Geometry: final body of the model. Coordinates: model frame, mm. Round coordinates to 2 decimals unless told otherwise and drop trailing zeros. Loops run counter-clockwise (first coordinate to the right, second up) from the corner with the lowest first, then second, coordinate; pieces in that order, holes last. Notation, with made-up numbers: (8.5, 38.25) - (36.5, 38.25) arc R16 cw to (36.5, 52.25) - close; hole circle Ø6 at (78.25, 33). An arc over 180 degrees is marked (long way). Answer in a Markdown table with one row per item. Add a question column.
from build123d import *

# Parameters (mm, degrees)
ESQUISSE1_R             = 47.5
BOSS_EXTRU_1_DEPTH      = 10
ESQUISSE3_W             = 100
ESQUISSE3_H             = 10
ENL_V_MAT_EXTRU_1_DEPTH = 11
ESQUISSE4_R             = 2.5
ENL_V_MAT_EXTRU_2_DEPTH = 11
ESQUISSE6_W             = 150
ESQUISSE6_H             = 120
BOSS_EXTRU_2_DEPTH      = 10
ESQUISSE7_W             = 10
ESQUISSE7_H             = 50
ESQUISSE7_W_2           = 50
ESQUISSE7_H_2           = 9.570800355
ENL_V_MAT_EXTRU_3_DEPTH = 10


with BuildPart() as part:
    # Esquisse1 → Boss.-Extru.1 (new body)
    with BuildSketch(Plane.XY):
        Polygon((-310, -75.642859016), (0, 414.561180135), (310, -75.642859016), align=None)
        with Locations((-157.5, 0)):
            Circle(ESQUISSE1_R, mode=Mode.SUBTRACT)
        with Locations((-52.5, 0)):
            Circle(ESQUISSE1_R, mode=Mode.SUBTRACT)
        with Locations((52.5, 0)):
            Circle(ESQUISSE1_R, mode=Mode.SUBTRACT)
        with Locations((157.5, 0)):
            Circle(ESQUISSE1_R, mode=Mode.SUBTRACT)
        with Locations((-105, 90.932667397)):
            Circle(ESQUISSE1_R, mode=Mode.SUBTRACT)
        with Locations((0, 90.932667397)):
            Circle(ESQUISSE1_R, mode=Mode.SUBTRACT)
        with Locations((105, 90.932667397)):
            Circle(ESQUISSE1_R, mode=Mode.SUBTRACT)
        with Locations((-52.5, 181.865334795)):
            Circle(ESQUISSE1_R, mode=Mode.SUBTRACT)
        with Locations((52.5, 181.865334795)):
            Circle(ESQUISSE1_R, mode=Mode.SUBTRACT)
        with Locations((0, 272.798002192)):
            Circle(ESQUISSE1_R, mode=Mode.SUBTRACT)
    extrude(amount=BOSS_EXTRU_1_DEPTH)

    # Esquisse3 → Enlèv. mat.-Extru.1 (cut, through all)
    with BuildSketch(Plane.XY.offset(10)):
        Polygon((-269.913793103, -12.254405678), (-261.461999325, -17.599233264), (-208.013723463, 66.918704521), (-216.465517241, 72.263532107), align=None)
        Polygon((-181.724137931, 127.200191667), (-173.272344153, 121.855364081), (-119.82406829, 206.373301865), (-128.275862069, 211.718129452), align=None)
        Polygon((-93.534482759, 266.654789012), (-85.08268898, 261.309961425), (-31.634413118, 345.82789921), (-40.086206897, 351.172726796), align=None)
        Polygon((269.913793103, -12.254405678), (261.461999325, -17.599233264), (208.013723463, 66.918704521), (216.465517241, 72.263532107), align=None)
        Polygon((181.724137931, 127.200191667), (173.272344153, 121.855364081), (119.82406829, 206.373301865), (128.275862069, 211.718129452), align=None)
        Polygon((93.534482759, 266.654789012), (85.08268898, 261.309961425), (31.634413118, 345.82789921), (40.086206897, 351.172726796), align=None)
        with Locations((-160, -70.642859016)):
            Rectangle(ESQUISSE3_W, ESQUISSE3_H)
        with Locations((160, -70.642859016)):
            Rectangle(ESQUISSE3_W, ESQUISSE3_H)
    extrude(amount=-ENL_V_MAT_EXTRU_1_DEPTH, mode=Mode.SUBTRACT)

    # Esquisse4 → Enlèv. mat.-Extru.2 (cut, through all)
    with BuildSketch(Plane.XY.offset(10)):
        with Locations((-157.5, -55.642859016)):
            Circle(ESQUISSE4_R)
        with Locations((-52.5, -55.642859016)):
            Circle(ESQUISSE4_R)
        with Locations((52.5, -55.642859016)):
            Circle(ESQUISSE4_R)
        with Locations((157.5, -55.642859016)):
            Circle(ESQUISSE4_R)
        with Locations((-105, 29.047375097)):
            Circle(ESQUISSE4_R)
        with Locations((0, 29.047375097)):
            Circle(ESQUISSE4_R)
        with Locations((105, 29.047375097)):
            Circle(ESQUISSE4_R)
        with Locations((-52.5, 119.980042494)):
            Circle(ESQUISSE4_R)
        with Locations((52.5, 119.980042494)):
            Circle(ESQUISSE4_R)
        with Locations((0, 210.912709891)):
            Circle(ESQUISSE4_R)
    extrude(amount=-ENL_V_MAT_EXTRU_2_DEPTH, mode=Mode.SUBTRACT)

    # Esquisse6 → Boss.-Extru.2 (add)
    with BuildSketch(Plane.XY.offset(10)):
        with Locations((0, -135.642859016)):
            Rectangle(ESQUISSE6_W, ESQUISSE6_H)
    extrude(amount=-BOSS_EXTRU_2_DEPTH)

    # Esquisse7 → Enlèv. mat.-Extru.3 (cut)
    with BuildSketch(Plane.XY.offset(10)):
        with Locations((-70, -135.642859016)):
            Rectangle(ESQUISSE7_W, ESQUISSE7_H)
        with Locations((0, -190.857458839)):
            Rectangle(ESQUISSE7_W_2, ESQUISSE7_H_2)
        with Locations((70, -135.642859016)):
            Rectangle(ESQUISSE7_W, ESQUISSE7_H)
    extrude(amount=-ENL_V_MAT_EXTRU_3_DEPTH, mode=Mode.SUBTRACT)


solid = part.part
1) Section D-D, the plane y = 373.5. Return the cut outline in (x, z).
2) Section A-A, the plane y = 0. Return the cut outline in (x, z).
3) Pull-direction query (Y, two-part tool) for faces 1 (the flat face through (1, 20, 10)), 2 (the flat face through (198.85, 100.12, 4.93)), 3 (the cylindrical face through (147.2, -46.37, 4.93)), 4 (the cylindrical face through (-10.297, 44.562, 4.93)); classes: pulls with the +Y half, pulls with the -Y half, needs draft (parallel to the pull), parting line crosses it, or undercut.
4) Contact query for flat-ended pins moving along their axis: pin 1 Ø5 at (x, z) = (235.5, 5.5) entering from -Y; pin 2 Ø5 at (x, z) = (-123.5, 4.5) entering from -Y; pin 3 Ø3 at (y, z) = (-72.5, 6.5) entering from -X. Output: stop coordinate, or through.
5) Material intervals for line 1 along X through (y, z) = (-74, 7); line 2 along Y through (x, z) = (-122, 6.25); line 3 along Y through (x, z) = (-52.5, 3), sorted ascending. Write a range as from..to.
6) Section B-B, the plane y = 194.5. Return the cut outline in (x, z).
7) Section C-C, the plane y = -91. Return the cut outline in (x, z), and give its area (3 significant figures).
Evaluation:
| question | item | result |
|---|---|---|
| 1 | outline | (-25.97, 0) - (25.97, 0) - (25.97, 10) - (-25.97, 10) - close |
| 2 | outline | (-250.33, 0) - (-205, 0) - (-205, 10) - (-250.33, 10) - close; (-110, 0) - (-100, 0) - (-100, 10) - (-110, 10) - close; (-5, 0) - (5, 0) - (5, 10) - (-5, 10) - close; (100, 0) - (110, 0) - (110, 10) - (100, 10) - close; (205, 0) - (250.33, 0) - (250.33, 10) - (205, 10) - close |
| 3 | face 1 | needs draft |
| 3 | face 2 | pulls with the +Y half |
| 3 | face 3 | undercut |
| 3 | face 4 | undercut |
| 4 | pin 1 | stops at y = -75.64 |
| 4 | pin 2 | stops at y = -65.64 |
| 4 | pin 3 | stops at x = -308.96 |
| 5 | line 1 | x = -308.96..-210, -110..110, 210..308.96 |
| 5 | line 2 | y = -65.64..-31.56, 31.56..46.58, 135.29..202.93, 207.75..221.64 |
| 5 | line 3 | y = -195.64..-58.14, -53.14..-47.5, 47.5..117.48, 122.48..134.37, 229.37..312.83 |
| 6 | outline | (-127.33, 0) - (-98.29, 0) - (-98.29, 10) - (-127.33, 10) - close; (-6.71, 0) - (6.71, 0) - (6.71, 10) - (-6.71, 10) - close; (98.29, 0) - (127.33, 0) - (127.33, 10) - (98.29, 10) - close |
| 7 | outline | (-75, 0) - (75, 0) - (75, 10) - (-75, 10) - close |
| 7 | area | 1,500 mm² |
